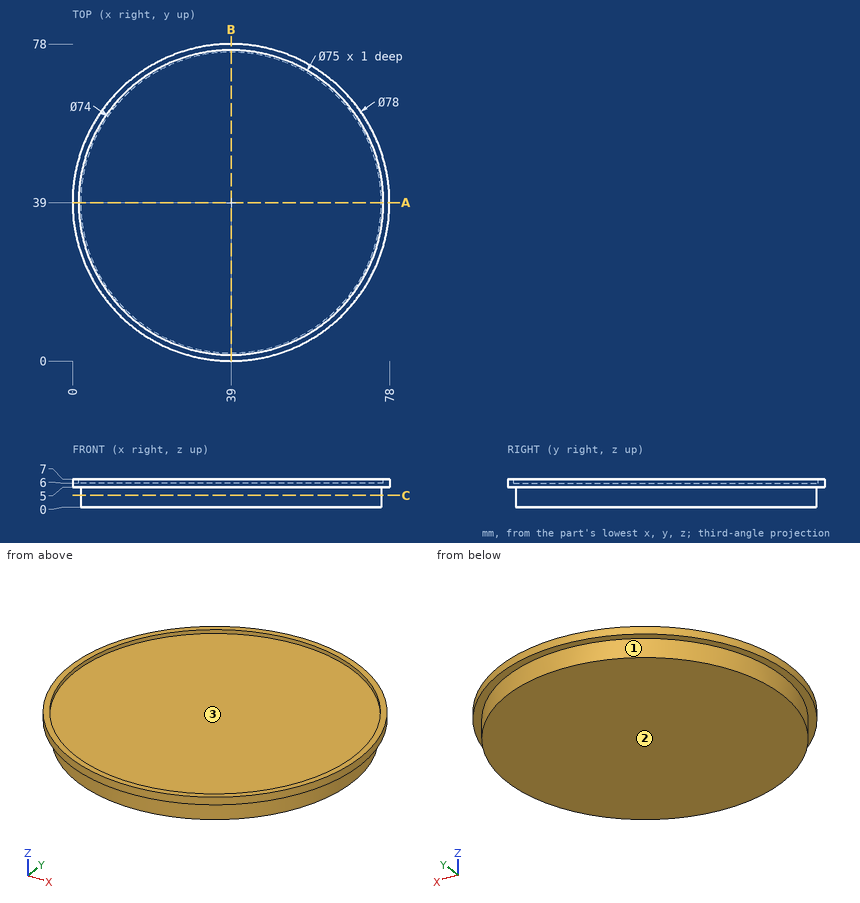
Could you check a few things on this drawing? It's one solid part, dimensions in mm from its lowest x, y, z. A direction names the side the tool comes from. Give positions to 0.01 mm unless a question says otherwise; leave off trailing zeros. Loops run counter-clockwise (first coordinate to the right, second up) from the corner with the lowest first, then second, coordinate; pieces in that order, holes last. Notation, with made-up numbers: M 25,1 L 84,1 A14 ccw 84,5 Z; hole C -13,0.25 d10. An arc over 180 degrees is marked long. One line per question, with ' | ' between items. Start each with the question number.
Q1. For pin 1 Ø1.5 at (y, z) = (20, 1) entering from +X; pin 2 Ø2 at (x, z) = (19.5, 6) entering from +Y; pin 3 Ø5 at (x, y) = (59, 64.5) entering from +Z, each with a flat end and sliding along its axis, tell me the tip position at first contact or that it passes through.
Q2. For the marked faces 1, 2 and 3, which set-ups out of +Z, -Z, +X, -X, +Y, -Y let a thin tool reach every point of the face, with its end or its side?
Q3. If we section it at A-A (y = 39): Please give me the cut outline in (x, z).
Q4. If we section it at C-C (z = 3): Please give me the cut outline in (x, y).
Q5. If I drill on line 1 (X direction, y = 39, z = 6.4); line 2 (Z direction, x = 71, y = 17); line 3 (Z direction, x = 61, y = 19.5), over which ranges is the centre line in solid material (lowest first)? Write a range as from..to.
Computed:
1) pin 1: stops at x = 71.19 | pin 2: stops at y = 73.33 | pin 3: stops at z = 6
2) face 1: -Z | face 2: -Z, +X, -X, +Y, -Y | face 3: +Z
3) outline: M 0,5 L 2,5 L 2,0 L 76,0 L 76,5 L 78,5 L 78,7 L 76.5,7 L 76.5,6 L 1.5,6 L 1.5,7 L 0,7 Z
4) outline: C 39,39 d74
5) line 1: x = 0..1.5, 76.5..78 | line 2: z = 5..7 | line 3: z = 0..6
